from build123d import *

# Parameters (mm, degrees)
F0_W     = 419.1
F0_H     = 76.2
F1_DEPTH = 6.35
F2_W     = 6.35
F2_H     = 6.35
F2_H_2   = 12.7
F2_H_3   = 31.75
F3_DEPTH = 6.35
F4_W     = 27.214286
F4_H     = 6.35
F4_W_2   = 27.214285
F4_W_3   = 6.35
F5_DEPTH = 6.351
F6_W     = 6.35
F6_H     = 12.7
F7_DEPTH = 6.351


with BuildPart() as f1:
    # F0 (on Front) → F1 (new body)
    with BuildSketch(Plane.XZ):
        with Locations((209.55, 38.1)):
            Rectangle(F0_W, F0_H)
    extrude(amount=F1_DEPTH)

    # F2 (on face) → F3 (cut, through all)
    with BuildSketch(Plane.XZ.offset(6.35)):
        with Locations((3.175, 3.175)):
            Rectangle(F2_W, F2_H)
        with Locations((3.175, 69.85)):
            Rectangle(F2_W, F2_H_2)
        with Locations((3.175, 34.925)):
            Rectangle(F2_W, F2_H_3)
        with Locations((415.925, 3.175)):
            Rectangle(F2_W, F2_H)
        with Locations((415.925, 34.925)):
            Rectangle(F2_W, F2_H_3)
        with Locations((415.925, 69.85)):
            Rectangle(F2_W, F2_H_2)
    extrude(amount=-F3_DEPTH, mode=Mode.SUBTRACT)

    # F4 (on face) → F5 (cut, through all)
    with BuildSketch(Plane.XZ.offset(6.35)):
        with Locations((51.707143, 3.175)):
            Rectangle(F4_W, F4_H)
        with Locations((104.321428, 3.175)):
            Rectangle(F4_W_2, F4_H)
        with Locations((156.935714, 3.175)):
            Rectangle(F4_W, F4_H)
        with Locations((209.55, 3.175)):
            Rectangle(F4_W, F4_H)
        with Locations((262.164286, 3.175)):
            Rectangle(F4_W, F4_H)
        with Locations((314.778571, 3.175)):
            Rectangle(F4_W_2, F4_H)
        with Locations((367.392857, 3.175)):
            Rectangle(F4_W, F4_H)
        with Locations((9.525, 3.175)):
            Rectangle(F4_W_3, F4_H)
        with Locations((409.575, 3.175)):
            Rectangle(F4_W_3, F4_H)
    extrude(amount=-F5_DEPTH, mode=Mode.SUBTRACT)

    # F6 (on face) → F7 (cut, through all)
    with BuildSketch(Plane.XZ.offset(6.35)):
        with Locations((85.725, 12.7)):
            Rectangle(F6_W, F6_H)
        with Locations((85.725, 57.15)):
            Rectangle(F6_W, F6_H)
        with Locations((333.375, 57.15)):
            Rectangle(F6_W, F6_H)
        with Locations((333.375, 12.7)):
            Rectangle(F6_W, F6_H)
        with Locations((168.275, 57.15)):
            Rectangle(F6_W, F6_H)
        with Locations((168.275, 12.7)):
            Rectangle(F6_W, F6_H)
        with Locations((250.825, 57.15)):
            Rectangle(F6_W, F6_H)
        with Locations((250.825, 12.7)):
            Rectangle(F6_W, F6_H)
    extrude(amount=-F7_DEPTH, mode=Mode.SUBTRACT)


solid = f1.part
Model file for the job. Use its own axes, mm. Coordinates: 2 decimals unless noted, no trailing zeros. Loops run counter-clockwise (first coordinate to the right, second up) from the corner with the lowest first, then second, coordinate; pieces in that order, holes last. Notation, with made-up numbers: (-36.5, 29.25) -> (-19.5, 29.25) arc R19 cw to (-19.5, 46.25) -> close; hole circle Ø9 at (80.5, 44.25). An arc over 180 degrees is marked (long way). Use one line per item in the form item = value. Start each with the question number.
(1) Cut at A-A on z = 13.5. Give the cut face in (x, y), and give its area (3 significant figures).
(2) Probe probe 1 along X at (y, z) = (-3.5, 9.5); probe 2 along Z at (x, y) = (311, -3); probe 3 along X at (y, z) = (-2, 21.5). List the from-to ranges inside material, lowest first. Write a range as from..to.
(3) Cut at B-B on y = -3. Give the number of separate pieces and of enclosed holes in the cut face, and give its area (3 significant figures).
(4) Cut at C-C on x = 219. Give the cut face in (y, z), and give its area (3 significant figures).
(5) Flat gauge pins, fed straight in: pin 1 (1.9 mm diameter, centred on y = -3, z = 3, fed in from -X); pin 2 (1.9 mm diameter, centred on y = -3.5, z = 29.5, fed in from +X); pin 3 (3 mm diameter, centred on x = 367, y = -4.5, fed in from -Z). Where does each tip first touch, or does it go through?
(6) Cut at D-D on z = 40.5. Give the cut face in (x, y), and give its area (3 significant figures).
Values:
q1.outline = (0, -6.35) -> (82.55, -6.35) -> (82.55, 0) -> (0, 0) -> close; (88.9, -6.35) -> (165.1, -6.35) -> (165.1, 0) -> (88.9, 0) -> close; (171.45, -6.35) -> (247.65, -6.35) -> (247.65, 0) -> (171.45, 0) -> close; (254, -6.35) -> (330.2, -6.35) -> (330.2, 0) -> (254, 0) -> close; (336.55, -6.35) -> (419.1, -6.35) -> (419.1, 0) -> (336.55, 0) -> close
q1.area = 2,500 mm2
q2.probe_1 = 0..82.55, 88.9..165.1, 171.45..247.65, 254..330.2, 336.55..419.1
q2.probe_2 = 6.35..76.2
q2.probe_3 = 6.35..412.75
q3.separate_pieces = 1
q3.enclosed_holes = 6
q3.area = 29,400 mm2
q4.outline = (-6.35, 6.35) -> (0, 6.35) -> (0, 76.2) -> (-6.35, 76.2) -> close
q4.area = 444 mm2
q5.pin_1 = 12.7
q5.pin_2 = 412.75
q5.pin_3 = 6.35
q6.outline = (6.35, -6.35) -> (412.75, -6.35) -> (412.75, 0) -> (6.35, 0) -> close
q6.area = 2,580 mm2
